```python
from build123d import *

# Parameters (mm, degrees)
BOSS_EXTRUDE1_DEPTH = 3
BOSS_EXTRUDE2_DEPTH = 2
SKETCH3_R           = 2.5
CUT_EXTRUDE1_DEPTH  = 3
SKETCH4_R           = 1.5
CUT_EXTRUDE2_DEPTH  = 10
SKETCH5_R           = 2.5
CUT_EXTRUDE3_DEPTH  = 4
SKETCH6_R           = 2.5
CUT_EXTRUDE6_DEPTH  = 188.014816174


with BuildPart() as part:
    # Sketch1 → Boss-Extrude1 (new body)
    with BuildSketch(Plane(origin=(0, 0, 0), x_dir=(1, 0, 0), z_dir=(0, 1, 0))):
        Polygon((-72.724629944, 121.633442715), (117.275370056, 121.633442715), (142.024107398, 96.884705373), (142.024107398, -93.115294627), (117.275370056, -117.864031968), (-72.724629944, -117.864031968), (-97.473367285, -93.115294627), (-97.473367285, 96.884705373), align=None)
    extrude(amount=BOSS_EXTRUDE1_DEPTH)

    # Sketch2 → Boss-Extrude2 (add)
    with BuildSketch(Plane(origin=(0, 3, 0), x_dir=(1, 0, 0), z_dir=(0, 1, 0))):
        Polygon((-97.473367285, -93.115294627), (-58.58249432, -54.224421662), (-33.833756978, -78.973159003), (-72.724629944, -117.864031968), align=None)
        Polygon((142.024107398, -93.115294627), (106.643904841, -53.574025356), (80.60097798, -76.876363508), (117.275370056, -117.864031968), align=None)
        Polygon((117.275370056, 121.633442715), (77.827961767, 85.647210429), (101.391526244, 59.817289105), (142.024107398, 96.884705373), align=None)
        Polygon((-72.724629944, 121.633442715), (-36.009112401, 80.682609127), (-62.030072457, 57.352851665), (-97.473367285, 96.884705373), align=None)
    extrude(amount=-BOSS_EXTRUDE2_DEPTH)

    # Sketch3 → Cut-Extrude1 (cut)
    with BuildSketch(Plane(origin=(0, 3, 0), x_dir=(1, 0, 0), z_dir=(0, 1, 0))):
        with Locations(Location((134.953039586, -82.508692909, 0), (0, 0, 270))):
            Circle(SKETCH3_R)
        with Locations(Location((106.668768338, -110.792964157, 0), (0, 0, 270))):
            Circle(SKETCH3_R)
        with Locations(Location((85.455564903, -89.579760721, 0), (0, 0, 270))):
            Circle(SKETCH3_R)
        with Locations(Location((113.73983615, -61.295489474, 0), (0, 0, 270))):
            Circle(SKETCH3_R)
        with Locations(Location((106.668768338, 114.562374903, 0), (0, 0, 270))):
            Circle(SKETCH3_R)
        with Locations(Location((134.953039586, 86.278103655, 0), (0, 0, 270))):
            Circle(SKETCH3_R)
        with Locations(Location((113.73983615, 65.06490022, 0), (0, 0, 270))):
            Circle(SKETCH3_R)
        with Locations(Location((85.455564903, 93.349171467, 0), (0, 0, 270))):
            Circle(SKETCH3_R)
        with Locations(Location((-62.118028226, 114.562374903, 0), (0, 0, 270))):
            Circle(SKETCH3_R)
        with Locations(Location((-90.402299473, 86.278103655, 0), (0, 0, 270))):
            Circle(SKETCH3_R)
        with Locations(Location((-69.189096038, 65.06490022, 0), (0, 0, 270))):
            Circle(SKETCH3_R)
        with Locations(Location((-40.90482479, 93.349171467, 0), (0, 0, 270))):
            Circle(SKETCH3_R)
        with Locations(Location((-40.90482479, -89.579760721, 0), (0, 0, 270))):
            Circle(SKETCH3_R)
        with Locations(Location((-69.189096038, -61.295489474, 0), (0, 0, 270))):
            Circle(SKETCH3_R)
        with Locations(Location((-62.118028226, -110.792964157, 0), (0, 0, 270))):
            Circle(SKETCH3_R)
        with Locations(Location((-90.402299473, -82.508692909, 0), (0, 0, 270))):
            Circle(SKETCH3_R)
    extrude(amount=-CUT_EXTRUDE1_DEPTH, mode=Mode.SUBTRACT)

    # Sketch4 → Cut-Extrude2 (cut)
    with BuildSketch(Plane(origin=(0, 3, 0), x_dir=(1, 0, 0), z_dir=(0, 1, 0))):
        with Locations(Location((39.275370056, -15.115294627, 0), (0, 0, 270))):
            Circle(SKETCH4_R)
        with Locations(Location((45.275370056, -21.115294627, 0), (0, 0, 270))):
            Circle(SKETCH4_R)
        with Locations(Location((39.275370056, 18.884705373, 0), (0, 0, 270))):
            Circle(SKETCH4_R)
        with Locations(Location((45.275370056, 24.884705373, 0), (0, 0, 270))):
            Circle(SKETCH4_R)
        with Locations(Location((5.275370056, 18.884705373, 0), (0, 0, 270))):
            Circle(SKETCH4_R)
        with Locations(Location((-0.724629944, 24.884705373, 0), (0, 0, 270))):
            Circle(SKETCH4_R)
        with Locations(Location((5.275370056, -15.115294627, 0), (0, 0, 270))):
            Circle(SKETCH4_R)
        with Locations(Location((-0.724629944, -21.115294627, 0), (0, 0, 270))):
            Circle(SKETCH4_R)
    extrude(amount=-CUT_EXTRUDE2_DEPTH, mode=Mode.SUBTRACT)

    # Sketch5 → Cut-Extrude3 (cut)
    with BuildSketch(Plane(origin=(0, 3, 0), x_dir=(1, 0, 0), z_dir=(0, 1, 0))):
        with Locations(Location((-65.653562132, 89.813637561, 0), (0, 0, 270))):
            Circle(SKETCH5_R)
        with Locations(Location((110.204302244, 89.813637561, 0), (0, 0, 270))):
            Circle(SKETCH5_R)
        with Locations(Location((110.204302244, -86.044226815, 0), (0, 0, 270))):
            Circle(SKETCH5_R)
        with Locations(Location((-65.653562132, -86.044226815, 0), (0, 0, 270))):
            Circle(SKETCH5_R)
    extrude(amount=-CUT_EXTRUDE3_DEPTH, mode=Mode.SUBTRACT)

    # Sketch6 → Cut-Extrude6 (cut, through all)
    with BuildSketch(Plane(origin=(0, 3, 0), x_dir=(1, 0, 0), z_dir=(0, 1, 0))):
        with Locations(Location((-63.224629944, -47.115294627, 0), (0, 0, 270))):
            Circle(SKETCH6_R)
        with Locations(Location((-63.224629944, 50.884705373, 0), (0, 0, 270))):
            Circle(SKETCH6_R)
        with Locations(Location((107.775370056, 50.884705373, 0), (0, 0, 270))):
            Circle(SKETCH6_R)
        with Locations(Location((107.775370056, -47.115294627, 0), (0, 0, 270))):
            Circle(SKETCH6_R)
        with Locations(Location((61.275370056, -47.115294627, 0), (0, 0, 270))):
            Circle(SKETCH6_R)
        with Locations(Location((22.275370056, -47.115294627, 0), (0, 0, 270))):
            Circle(SKETCH6_R)
        with Locations(Location((-16.724629944, -47.115294627, 0), (0, 0, 270))):
            Circle(SKETCH6_R)
        with Locations(Location((-16.724629944, 50.884705373, 0), (0, 0, 270))):
            Circle(SKETCH6_R)
        with Locations(Location((22.275370056, 50.884705373, 0), (0, 0, 270))):
            Circle(SKETCH6_R)
        with Locations(Location((61.275370056, 50.884705373, 0), (0, 0, 270))):
            Circle(SKETCH6_R)
    extrude(amount=-CUT_EXTRUDE6_DEPTH, mode=Mode.SUBTRACT)


solid = part.part
```
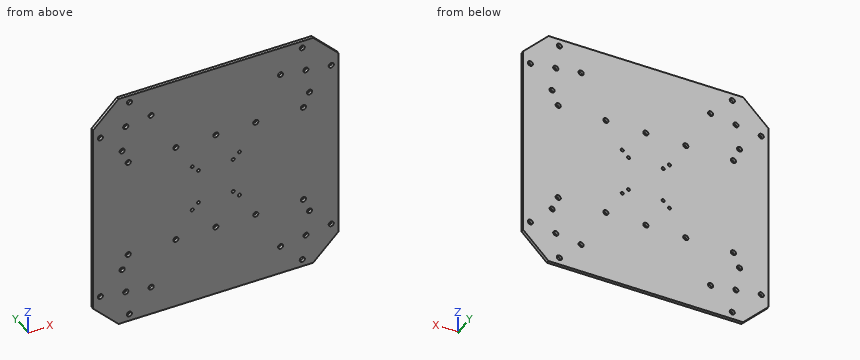
Can you work these out from the model? Positions are in its coordinate system, mm. Round coordinates to 2 decimals unless told otherwise and drop trailing zeros. Loops run counter-clockwise (first coordinate to the right, second up) from the corner with the lowest first, then second, coordinate; pieces in that order, holes last. Notation, with made-up numbers: M 64,-23.75 L 93,-23.75 A14 cw 93,-15.75 Z; hole C 5,75.25 d4. An arc over 180 degrees is marked long. Answer as a JSON object with one key per item and string values. Group by question number.
Q1. Imagine slicing it at A-A, the plane z = -106.5. Please give me the cut outline in (x, y).
Q2. Imagine slicing it at B-B, the plane y = 1.15. Count the separate pieces of the cut face and the enclosed holes in it, then the cut area to 3 significant figures.
Q3. Please list where these lines run through material, in increasing order: L1, parallel to X at y = 2.65, z = 83; L2, parallel to Z at x = -66, y = 1.8; L3, parallel to X at y = 2.55, z = -51.
Q4. Imagine slicing it at C-C, the plane x = 124.5. Please give me the cut outline in (y, z), then the cut area to 3 significant figures.
Findings:
{
 "1": {"outline": "M -87.86,0 L 132.41,0 L 132.41,3 L -87.86,3 Z"},
 "2": {"separate pieces": "1", "enclosed holes": "38", "area": "55,500 mm2"},
 "3": {"L1": "x = -97.47 to -92.85, -87.95 to 132.5, 137.4 to 142.02", "L2": "z = -121.63 to -92.29, -87.34 to 83.57, 88.52 to 117.86", "L3": "x = -97.47 to -65.72, -60.73 to -19.22, -14.23 to 19.78, 24.77 to 58.78, 63.77 to 105.28, 110.27 to 142.02"},
 "4": {"outline": "M 0,-114.41 L 3,-114.41 L 3,110.64 L 0,110.64 Z", "area": "675 mm2"}
}
